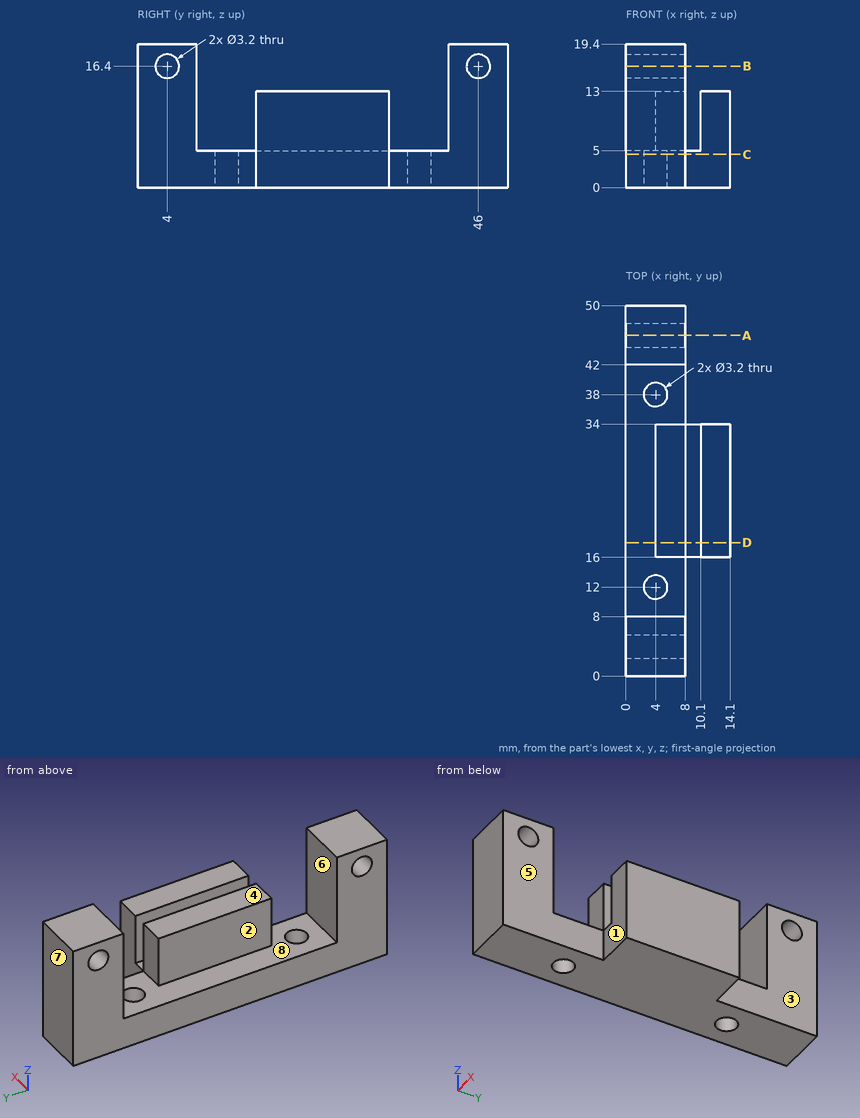
Geometry: see drawing. Coordinates: mm, zero at the bounding-box minimum. A direction names the side the tool comes from. Give positions to 0.01 mm unless a question says otherwise; leave off trailing zeros. Loops run counter-clockwise (first coordinate to the right, second up) from the corner with the lowest first, then second, coordinate; pieces in that order, holes last. Notation, with made-up numbers: M 19,86 L 51,86 A22 ccw 51,118 Z; hole C -33.75,-15.75 d10. An arc over 180 degrees is marked long. Use one line per item in the form item = value.
1. Section query D-D, the plane y = 18. Return the cut outline in (x, z), and give its area (4 significant figures).
Numbers:
outline = M 0,0 L 14.1,0 L 14.1,13 L 10.1,13 L 10.1,5 L 8,5 L 8,13 L 4,13 L 4,5 L 0,5 Z
area = 134.5 mm²
2. Section query A-A, the plane y = 46. Return the cut outline in (x, z), and give its area (3 significant figures).
Numbers:
outline = M 0,0 L 8,0 L 8,14.8 L 0,14.8 Z; M 0,18 L 8,18 L 8,19.4 L 0,19.4 Z
area = 130 mm²
3. Pull-direction query (Y, two-part tool) for the marked faces 5, 6, 7 and 8; classes: released by +Y, released by -Y, zero draft, split by the parting line, or undercut.
Numbers:
face_5 = zero draft
face_6 = undercut
face_7 = released by +Y
face_8 = undercut
4. Line query: L1, parallel to Y at x = 1.75, z = 16.4; L2, parallel to Y at x = 4, z = 2.7; L3, parallel to Y at x = 4.75, z = 7.5. Output: solid intervals per line, ascending.
Numbers:
L1 = 0 to 2.4, 5.6 to 8, 42 to 44.4, 47.6 to 50
L2 = 0 to 10.4, 13.6 to 36.4, 39.6 to 50
L3 = 0 to 8, 16 to 34, 42 to 50
5. First-contact query: pin 1 (2.5 mm diameter, centred on x = 2, y = 26, fed in from +Z); pin 2 (2.5 mm diameter, centred on x = 8.5, y = 24.5, fed in from +Z); pin 3 (4 mm diameter, centred on y = 25, z = 8, fed in from -X). Flat tips, straight axial feed; report the tip coordinate or a pass-through.
Numbers:
pin_1 = 5
pin_2 = 13
pin_3 = 4
6. Section query B-B, the plane z = 16.4. Return the cut outline in (x, y), and give its area (3 significant figures).
Numbers:
outline = M 0,0 L 8,0 L 8,2.4 L 0,2.4 Z; M 0,5.6 L 8,5.6 L 8,8 L 0,8 Z; M 0,42 L 8,42 L 8,44.4 L 0,44.4 Z; M 0,47.6 L 8,47.6 L 8,50 L 0,50 Z
area = 76.8 mm²
7. Reachability of the marked faces 1, 2, 3 and 4 from +Z, -Z, +X, -X, +Y, -Y: full face, straight path, thin tool, end or side. Return the list, or none.
Numbers:
face_1 = +Z, -Z, +X, -Y
face_2 = +Z, -X
face_3 = +Z, -Z, +X, +Y
face_4 = +Z, +X, -X
8. Section query C-C, the plane z = 4.5. Return the cut outline in (x, y).
Numbers:
outline = M 0,0 L 8,0 L 8,16 L 14.1,16 L 14.1,34 L 8,34 L 8,50 L 0,50 Z; hole C 4,12 d3.2; hole C 4,38 d3.2
